Check sheet for the modelled part. Datum: model origin and axes. Units: mm. Face numbers are marked on the shaded views. A direction names the side the tool comes from. Coordinates: 2 decimals unless noted, no trailing zeros. Write each loop counter-clockwise with the first axis right and the second up, starting at its lowest first coordinate (ties: lowest second). Pieces come first, ordered by that corner, then holes. Notation, with made-up numbers: (-35.75, 16.25) - (-28.75, 16.25) arc R23 ccw to (-28.75, 54.25) - close; hole circle Ø10 at (-3.5, 74). An arc over 180 degrees is marked (long way). Use one line per item in the form item = value. Start each with the question number.
1. Cross-section at A-A on z = 15.25. Record the boundary of the cut face in (x, y), then the cut area to 3 significant figures.
2. Go/stop test with flat-tipped pins: pin 1 Ø3 at (x, y) = (-6.5, 4) entering from -Z; pin 2 Ø4 at (x, y) = (3, -2.5) entering from -Z; pin 3 Ø2 at (x, z) = (0, 25) entering from -Y; pin 4 Ø1.8 at (x, z) = (2, 25.5) entering from -Y. Record where each tip stops, or that it passes through.
3. Tool access check on the marked faces 1 and 2. Record the directions out of +Z, -Z, +X, -X, +Y, -Y that give a thin tool (end or side, any length) a straight path to the whole face; none if there is none.
4. Cross-section at D-D on z = 23.25. Record the boundary of the cut face in (x, y), then the cut area to 3 significant figures.
5. Cross-section at B-B on y = 0.5. Record the boundary of the cut face in (x, z), then the cut area to 3 significant figures.
6. Cross-section at C-C on y = -3.5. Record the boundary of the cut face in (x, z).
7. Scan lines: line 1 along X through (y, z) = (2.5, 15.25); line 2 along Z through (x, y) = (-4.5, 0.5); line 3 along X through (y, z) = (1.55, 23.25). Record each from-to range of solid material in increasing order.
8. Draft check along X on the marked faces 3, 4 and 5. Enter one of: +X half, -X half, draft (parallel to the pull), parting line (faces both ways), or undercut.
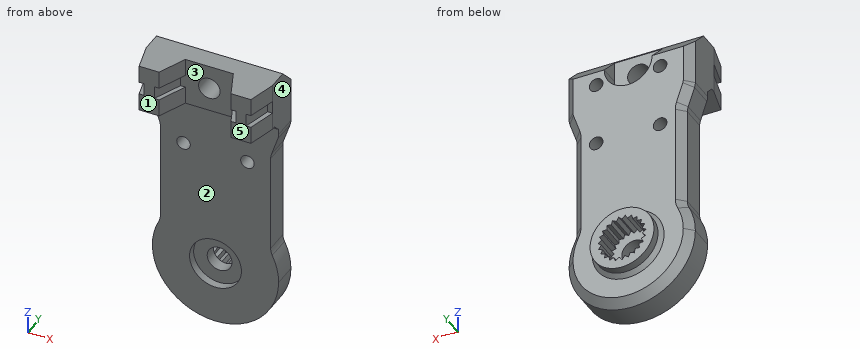
```python
from build123d import *
from build123d.topology import SkipClean

# Parameters (mm, degrees)
EXTRUDE_1_DEPTH          = 4
EXTRUDE_3_DEPTH          = 6
CHAMFER_1_SIZE           = 3
SKETCH_5_R               = 0.85
CUT_EXTRUDE_1_DEPTH      = 4
PATTERN_LINEAR_1_COUNT   = 2
PATTERN_LINEAR_1_PITCH   = 8
CUT_EXTRUDE_2_DEPTH      = 2.5
CUT_EXTRUDE_3_REACH      = 31.81
SKETCH_7_R               = 1.35
SKETCH_9_R               = 3.25
CUT_EXTRUDE_4_DEPTH      = 1
SKETCH_10_R              = 4
EXTRUDE_4_DEPTH          = 1.5
CHAMFER_3_SIZE           = 0.5
SKETCH_11_R              = 3
CUT_EXTRUDE_5_DEPTH      = 3
SKETCH_12_R              = 1.55
CUT_EXTRUDE_6_DEPTH      = 30.705386717
EXTRUDE_5_DEPTH          = 3
PATTERN_CIRCULAR_1_COUNT = 23
CUT_EXTRUDE_7_DEPTH      = 0.8
CUT_EXTRUDE_8_DEPTH      = 31.453407034
FILLET_1_R               = 2
CHAMFER_2_SIZE           = 1


with BuildPart() as part:
    # ｽｹｯﾁ1 → ﾎﾞｽ - 押し出し1 (new body)
    with BuildSketch(Plane(origin=(0, 0, 0), x_dir=(1, 0, 0), z_dir=(0, 1, 0))):
        with BuildLine():
            Line((-7.9, 0), (-7.9, -28))
            Line((-7.9, -28), (7.9, -28))
            Line((7.9, -28), (7.9, 0))
            ThreePointArc((7.9, 0), (0, 7.9), (-7.9, 0))
        make_face()
    extrude(amount=EXTRUDE_1_DEPTH)

    # ｽｹｯﾁ4 → ﾎﾞｽ - 押し出し3 (add)
    with BuildSketch(Plane.XY.offset(28)):
        Polygon((-7, -5), (-4.5, -5), (-3, -1.5), (3, -1.5), (4.5, -5), (7, -5), (7.9, -1.5), (7.9, 0), (-7.9, 0), (-7.9, -1.5), align=None)
    extrude(amount=-EXTRUDE_3_DEPTH)

    # 面取り1
    chamfer_1_edges = [part.edges().sort_by_distance(p)[0] for p in [
        (0, 4, 28),
    ]]
    chamfer(chamfer_1_edges, length=CHAMFER_1_SIZE)

    # ｽｹｯﾁ5 → ｶｯﾄ - 押し出し1 (cut)
    with BuildSketch(Plane(origin=(0, 4, 0), x_dir=(1, 0, 0), z_dir=(0, 1, 0))):
        with Locations(Location((-4, -23.25, 0), (0, 0, 270))):
            Circle(SKETCH_5_R)
        with Locations(Location((4, -23.25, 0), (0, 0, 270))):
            Circle(SKETCH_5_R)
    cut_extrude_1 = extrude(amount=-CUT_EXTRUDE_1_DEPTH, mode=Mode.SUBTRACT)

    # 直線ﾊﾟﾀｰﾝ1: ｶｯﾄ - 押し出し1 ×2
    with Locations(*[(0, 0, -i * PATTERN_LINEAR_1_PITCH) for i in range(1, PATTERN_LINEAR_1_COUNT)]):
        add(cut_extrude_1, mode=Mode.SUBTRACT)

    # ｽｹｯﾁ6 → ｶｯﾄ - 押し出し2 (cut)
    with BuildSketch(Plane(origin=(0, 4, 0), x_dir=(1, 0, 0), z_dir=(0, 1, 0))):
        with BuildLine():
            Line((-3, -25), (-3, -29))
            Line((-3, -29), (3, -29))
            Line((3, -29), (3, -25))
            ThreePointArc((3, -25), (0, -22), (-3, -25))
        make_face()
    extrude(amount=-CUT_EXTRUDE_2_DEPTH, mode=Mode.SUBTRACT)

    # ｽｹｯﾁ7 → ｶｯﾄ - 押し出し3 (cut, up to next)
    with BuildSketch(Plane(origin=(0, 1.5, 0), x_dir=(1, 0, 0), z_dir=(0, 1, 0)), mode=Mode.PRIVATE) as cut_extrude_3_sk1:
        with Locations(Location((0, -25, 0), (0, 0, 270))):
            Circle(SKETCH_7_R)
    cut_extrude_3_tool1 = extrude(cut_extrude_3_sk1.sketch, amount=-CUT_EXTRUDE_3_REACH, mode=Mode.PRIVATE) & part.part
    add(cut_extrude_3_tool1.solids().sort_by_distance((0, 1.5, 25))[0], mode=Mode.SUBTRACT)

    # ｽｹｯﾁ9 → ｶｯﾄ - 押し出し4 (cut)
    with BuildSketch(Plane(origin=(0, 0, 0), x_dir=(1, 0, 0), z_dir=(0, 1, 0))):
        with Locations(Location((0, 0, 0), (0, 0, 270))):
            Circle(SKETCH_9_R)
    extrude(amount=CUT_EXTRUDE_4_DEPTH, mode=Mode.SUBTRACT)

    # ｽｹｯﾁ10 → ﾎﾞｽ - 押し出し4 (add)
    with BuildSketch(Plane(origin=(0, 4, 0), x_dir=(1, 0, 0), z_dir=(0, 1, 0))):
        with Locations(Location((0, 0, 0), (0, 0, 270))):
            Circle(SKETCH_10_R)
    extrude(amount=EXTRUDE_4_DEPTH)

    # 面取り3
    chamfer_3_edges = [part.edges().sort_by_distance(p)[0] for p in [
        (0, 4, -4),
    ]]
    chamfer(chamfer_3_edges, length=CHAMFER_3_SIZE)

    # ｽｹｯﾁ11 → ｶｯﾄ - 押し出し5 (cut)
    with BuildSketch(Plane(origin=(0, 5.5, 0), x_dir=(1, 0, 0), z_dir=(0, 1, 0))):
        with Locations(Location((0, 0, 0), (0, 0, 270))):
            Circle(SKETCH_11_R)
    extrude(amount=-CUT_EXTRUDE_5_DEPTH, mode=Mode.SUBTRACT)

    # ｽｹｯﾁ12 → ｶｯﾄ - 押し出し6 (cut, through all)
    with BuildSketch(Plane.XZ.offset(-1)):
        with Locations(Location((0, 0, 0), (0, 0, 270))):
            Circle(SKETCH_12_R)
    extrude(amount=-CUT_EXTRUDE_6_DEPTH, mode=Mode.SUBTRACT)

    # ｽｹｯﾁ13 → ﾎﾞｽ - 押し出し5 (add)
    with BuildSketch(Plane(origin=(0, 5.5, 0), x_dir=(1, 0, 0), z_dir=(0, 1, 0))):
        with BuildLine():
            Line((0.408499947, -2.972057838), (0, -2.574530741))
            Line((0, -2.574530741), (-0.408499947, -2.972057838))
            ThreePointArc((-0.408499947, -2.972057838), (0, -3), (0.408499947, -2.972057838))
        make_face()
    extrude_5 = extrude(amount=-EXTRUDE_5_DEPTH)

    # 円形ﾊﾟﾀｰﾝ1: ﾎﾞｽ - 押し出し5 ×23 about axis
    pattern_circular_1_axis = Axis((0, 0, 0), (0, 1, 0))
    for i in range(1, PATTERN_CIRCULAR_1_COUNT):
        add(extrude_5.rotate(pattern_circular_1_axis, i * 360 / PATTERN_CIRCULAR_1_COUNT))

    # ｽｹｯﾁ14 → ｶｯﾄ - 押し出し7 (cut, symmetric)
    with BuildSketch(Plane.XY.offset(25)):
        Polygon((3, -1.5), (4.5, -5), (5.1, -5), (3.6, -1.5), align=None)
        Polygon((6.4, -5), (7, -5), (7.9, -1.5), (7.3, -1.5), align=None)
    cut_extrude_7 = extrude(amount=CUT_EXTRUDE_7_DEPTH, both=True, mode=Mode.SUBTRACT)

    # ﾐﾗｰ1: ｶｯﾄ - 押し出し7 across plane
    add(cut_extrude_7.mirror(Plane(origin=(0, 0, 0), x_dir=(0, 0, 1), z_dir=(1, 0, 0))), mode=Mode.SUBTRACT)

    # ｽｹｯﾁ15 → ｶｯﾄ - 押し出し8 (cut, through all)
    with SkipClean():  # the faces are left unmerged after this step: merging them gives an invalid solid
        with BuildSketch(Plane(origin=(0, 4, 0), x_dir=(1, 0, 0), z_dir=(0, 1, 0))):
            with BuildLine():
                Line((-7.9, 0), (-7.9, -20))
                Line((-7.9, -20), (-6.9, -17))
                Line((-6.9, -17), (-6.9, -3.847076812))
                ThreePointArc((-6.9, -3.847076812), (-7.645913941, -1.987460691), (-7.9, 0))
            make_face()
        cut_extrude_8 = extrude(amount=-CUT_EXTRUDE_8_DEPTH, mode=Mode.SUBTRACT)

    # ﾐﾗｰ2: ｶｯﾄ - 押し出し8 across plane
    with SkipClean():  # the faces are left unmerged after this step: merging them gives an invalid solid
        add(cut_extrude_8.mirror(Plane(origin=(0, 0, 0), x_dir=(0, 0, 1), z_dir=(1, 0, 0))), mode=Mode.SUBTRACT)

    # ﾌｨﾚｯﾄ1
    fillet_1_edges = [part.edges().sort_by_distance(p)[0] for p in [
        (-6.9, 2, 3.847076812),
        (-6.9, 2, 17),
        (-7.9, 2, 20),
        (6.9, 2, 3.847076812),
        (7.9, 2, 20),
        (6.9, 2, 17),
    ]]
    fillet(fillet_1_edges, radius=FILLET_1_R)

    # 面取り2
    chamfer_2_edges = [part.edges().sort_by_distance(p)[0] for p in [
        (-7.9, 4, 22.66227766),
        (0, 4, -7.9),
        (7.9, 4, 22.66227766),
        (0, 0, 22),
        (-7.874174915, 4, 20.004190834),
        (-7.4, 4, 18.5),
        (-6.925825085, 4, 16.995809166),
        (-6.9, 4, 10.505670679),
        (-6.951159371, 4, 3.886430103),
        (6.951159371, 4, 3.886430103),
        (6.9, 4, 10.505670679),
        (6.925825085, 4, 16.995809166),
        (7.4, 4, 18.5),
        (7.874174915, 4, 20.004190834),
    ]]
    chamfer(chamfer_2_edges, length=CHAMFER_2_SIZE)


solid = part.part
```
Final values:
q1.outline = (-6.9, 0) - (-4.85, 0) - (-4.85, 4) - (-5.9, 4) - (-6.9, 3) - close; (-3.15, 0) - (3.15, 0) - (3.15, 4) - (-3.15, 4) - close; (4.85, 0) - (6.9, 0) - (6.9, 3) - (5.9, 4) - (4.85, 4) - close
q1.area = 40.6 mm²
q2.pin_1 = -5.78
q2.pin_2 = 21.5
q2.pin_3 = through
q2.pin_4 = -1.5
q3.face_1 = +Z, -Z, +X, -X, -Y
q3.face_2 = -Z, +X, -X, -Y
q4.outline = (-7.9, -1.5) - (-7, -5) - (-4.5, -5) - (-3, -1.5) - (3, -1.5) - (4.5, -5) - (7, -5) - (7.9, -1.5) - (7.9, 3) - (6.9, 4) - (4.85, 4) - (4.85, 0) - (3.15, 0) - (3.15, 4) - (2.44, 4) - (2.44, 1.5) - (-2.44, 1.5) - (-2.44, 4) - (-3.15, 4) - (-3.15, 0) - (-4.85, 0) - (-4.85, 4) - (-6.9, 4) - (-7.9, 3) - close
q4.area = 86.0 mm²
q5.outline = (-7.9, 20.32) arc R2 ccw to (-7.8, 19.69) - (-7, 17.31) arc R2 cw to (-6.9, 16.68) - (-6.9, 4.34) arc R2 cw to (-7.1, 3.46) arc R7.9 ccw (long way) to (7.1, 3.46) arc R2 cw to (6.9, 4.34) - (6.9, 16.68) arc R2 cw to (7, 17.31) - (7.8, 19.69) arc R2 ccw to (7.9, 20.32) - (7.9, 28) - (-7.9, 28) - close; hole circle Ø1.7 at (-4, 15.25); hole circle Ø1.7 at (-4, 23.25); hole circle Ø6.5 at (0, 0); hole circle Ø2.7 at (0, 25); hole circle Ø1.7 at (4, 15.25); hole circle Ø1.7 at (4, 23.25)
q5.area = 461 mm²
q6.outline = (-7.39, 22) - (-3.86, 22) - (-3.86, 24.2) - (-4.46, 24.2) - (-4.46, 25.8) - (-3.86, 25.8) - (-3.86, 28) - (-7.39, 28) - (-7.39, 25.8) - (-6.79, 25.8) - (-6.79, 24.2) - (-7.39, 24.2) - close; (3.86, 22) - (7.39, 22) - (7.39, 24.2) - (6.79, 24.2) - (6.79, 25.8) - (7.39, 25.8) - (7.39, 28) - (3.86, 28) - (3.86, 25.8) - (4.46, 25.8) - (4.46, 24.2) - (3.86, 24.2) - close
q7.line_1 = -6.9 to -4.85, -3.15 to 3.15, 4.85 to 6.9
q7.line_2 = -6.49 to 14.56, 15.94 to 22.56, 23.94 to 28
q7.line_3 = -7.9 to -4.85, -3.15 to -2.44, 2.44 to 3.15, 4.85 to 7.9
q8.face_3 = undercut
q8.face_4 = +X half
q8.face_5 = draft
